Geometry check sheet. Reference: the model listing, model coordinates, mm. A direction names the side the tool comes from. Give positions to 0.01 mm unless a question says otherwise; leave off trailing zeros. Order: outer loops, then holes, each group sorted by start corner. A loop starts at its lowest first (then second) coordinate and runs counter-clockwise, first axis right, second up.
from build123d import *

# Parameters (mm, degrees)
SKETCH1_R                = 25
BOSS_EXTRUDE1_DEPTH      = 25
SKETCH9_W                = 25
SKETCH9_H                = 7.5
BOSS_EXTRUDE3_DEPTH      = 55
BOSS_EXTRUDE3_DEPTH_BACK = 55
SKETCH16_R               = 22.5
CUT_EXTRUDE3_DEPTH       = 7.5
SKETCH17_R               = 0.75
CUT_EXTRUDE4_DEPTH       = 10
SKETCH22_W               = 7.5
SKETCH22_H               = 25
BOSS_EXTRUDE7_DEPTH      = 30
SKETCH23_W               = 7.5
SKETCH23_H               = 60
BOSS_EXTRUDE8_DEPTH      = 110
SKETCH24_W               = 7.5
SKETCH24_H               = 80
BOSS_EXTRUDE9_DEPTH      = 110
SKETCH25_W               = 1.5
SKETCH25_H               = 110
BOSS_EXTRUDE10_DEPTH     = 2
SKETCH26_W               = 1.5
SKETCH26_H               = 110
BOSS_EXTRUDE11_DEPTH     = 2
FILLET6_R                = 5


with BuildPart() as part:
    # Sketch1 → Boss-Extrude1 (new body)
    with BuildSketch(Plane(origin=(0, 0, 0), x_dir=(1, 0, 0), z_dir=(0, 1, 0))):
        Circle(SKETCH1_R)
    extrude(amount=BOSS_EXTRUDE1_DEPTH)

    # Sketch9 → Boss-Extrude3 (add, two sides)
    with BuildSketch(Plane(origin=(0, 0, 0), x_dir=(0, 0, -1), z_dir=(1, 0, 0))) as boss_extrude3_sk:
        with Locations((0, 3.75)):
            Rectangle(SKETCH9_W, SKETCH9_H)
    extrude(amount=BOSS_EXTRUDE3_DEPTH)
    extrude(boss_extrude3_sk.sketch, amount=-BOSS_EXTRUDE3_DEPTH_BACK)

    # Sketch16 → Cut-Extrude3 (cut)
    with BuildSketch(Plane(origin=(0, 25, 0), x_dir=(1, 0, 0), z_dir=(0, 1, 0))):
        Circle(SKETCH16_R)
    extrude(amount=-CUT_EXTRUDE3_DEPTH, mode=Mode.SUBTRACT)

    # Sketch17 → Cut-Extrude4 (cut)
    with BuildSketch(Plane(origin=(0, 17.5, 0), x_dir=(1, 0, 0), z_dir=(0, 1, 0))):
        with BuildLine():
            ThreePointArc((-4, 3), (-3.535533906, 3.535533906), (-3, 4))
            Line((-3, 4), (-2, 22.410934831))
            ThreePointArc((-2, 22.410934831), (-15.909902577, 15.909902577), (-22.410934831, 2))
            Line((-22.410934831, 2), (-4, 3))
        make_face()
        with BuildLine():
            Line((2, 22.410934831), (3, 4))
            ThreePointArc((3, 4), (3.535533906, 3.535533906), (4, 3))
            Line((4, 3), (22.410934831, 2))
            ThreePointArc((22.410934831, 2), (15.909902577, 15.909902577), (2, 22.410934831))
        make_face()
        with BuildLine():
            ThreePointArc((-3, -4), (-3.535533906, -3.535533906), (-4, -3))
            Line((-4, -3), (-22.410934831, -2))
            ThreePointArc((-22.410934831, -2), (-15.909902577, -15.909902577), (-2, -22.410934831))
            Line((-2, -22.410934831), (-3, -4))
        make_face()
        with BuildLine():
            Line((22.410934831, -2), (4, -3))
            ThreePointArc((4, -3), (3.535533906, -3.535533906), (3, -4))
            Line((3, -4), (2, -22.410934831))
            ThreePointArc((2, -22.410934831), (15.909902577, -15.909902577), (22.410934831, -2))
        make_face()
        Circle(SKETCH17_R)
    extrude(amount=-CUT_EXTRUDE4_DEPTH, mode=Mode.SUBTRACT)

    # Sketch22 → Boss-Extrude7 (add)
    with BuildSketch(Plane.XZ):
        with Locations((-51.25, 0)):
            Rectangle(SKETCH22_W, SKETCH22_H)
    boss_extrude7 = extrude(amount=BOSS_EXTRUDE7_DEPTH)

    # Sketch23 → Boss-Extrude8 (add)
    with BuildSketch(Plane.XZ.offset(30)):
        with Locations((-51.25, 0)):
            Rectangle(SKETCH23_W, SKETCH23_H)
    extrude(amount=BOSS_EXTRUDE8_DEPTH)

    # Mirror1: Boss-Extrude7 across plane
    add(boss_extrude7.mirror(Plane(origin=(0, 0, 0), x_dir=(0, 0, 1), z_dir=(1, 0, 0))))

    # Sketch24 → Boss-Extrude9 (add)
    with BuildSketch(Plane.XZ.offset(30)):
        with Locations((51.25, 10)):
            Rectangle(SKETCH24_W, SKETCH24_H)
    extrude(amount=BOSS_EXTRUDE9_DEPTH)

    # Sketch25 → Boss-Extrude10 (add)
    with BuildSketch(Plane(origin=(-47.5, 0, 0), x_dir=(0, 0, -1), z_dir=(1, 0, 0))):
        with Locations((29.25, -85)):
            Rectangle(SKETCH25_W, SKETCH25_H)
    extrude(amount=BOSS_EXTRUDE10_DEPTH)

    # Sketch26 → Boss-Extrude11 (add)
    with BuildSketch(Plane.ZY.offset(-47.5)):
        with Locations((-29.25, -85)):
            Rectangle(SKETCH26_W, SKETCH26_H)
        with Locations((49.25, -85)):
            Rectangle(SKETCH26_W, SKETCH26_H)
    extrude(amount=BOSS_EXTRUDE11_DEPTH)

    # Fillet6
    fillet6_edges = [part.edges().sort_by_distance(p)[0] for p in [
        (-21.650635095, 3.75, 12.5),
        (21.650635095, 3.75, 12.5),
        (-55, 7.5, 0),
        (47.5, 0, 0),
        (21.650635095, 3.75, -12.5),
        (-21.650635095, 3.75, -12.5),
        (55, 7.5, 0),
        (-25, 7.5, 0),
        (-47.5, 0, 0),
        (24.148145657, 7.5, -6.470476128),
    ]]
    fillet(fillet6_edges, radius=FILLET6_R)


solid = part.part
Item 1: Scan lines: L1, parallel to X at y = -59, z = -1; L2, parallel to Z at x = 0, y = 12.75; L3, parallel to X at y = 10, z = 11. Record each from-to range of solid material in increasing order.
Reported:
L1: x = -55 to -47.5, 47.5 to 55
L2: z = -25 to -0.75, 0.75 to 25
L3: x = -23.19 to -19.63, -2.62 to 2.62, 19.63 to 23.19
Item 2: Sectioned sample at A-A (y = -77). Enter the section's corners in (x, z).
Reported:
outline: (-55, -30) - (-45.5, -30) - (-45.5, -28.5) - (-47.5, -28.5) - (-47.5, 30) - (-55, 30) - close; (45.5, -30) - (55, -30) - (55, 50) - (45.5, 50) - (45.5, 48.5) - (47.5, 48.5) - (47.5, -28.5) - (45.5, -28.5) - close
Item 3: Sectioned sample at D-D (y = 10). Enter the section's corners in (x, z), and give its area (3 significant figures).
Reported:
outline: (-22.11, -13.04) arc R5 cw to (-20.31, -14.58) arc R25 ccw to (20.31, -14.58) arc R5 cw to (22.11, -13.04) arc R25.67 ccw to (22.11, 13.04) arc R5 cw to (20.31, 14.58) arc R25 ccw to (-20.31, 14.58) arc R5 cw to (-22.11, 13.04) arc R25.67 ccw to start; hole (-22.41, -2) arc R22.5 ccw to (-2, -22.41) - (-3, -4) arc R5 cw to (-4, -3) - close; hole (-22.41, 2) - (-4, 3) arc R5 cw to (-3, 4) - (-2, 22.41) arc R22.5 ccw to start; hole circle Ø1.5 at (0, 0); hole (2, -22.41) arc R22.5 ccw to (22.41, -2) - (4, -3) arc R5 cw to (3, -4) - close; hole (2, 22.41) - (3, 4) arc R5 cw to (4, 3) - (22.41, 2) arc R22.5 ccw to start
area: 841 mm2
Item 4: Sectioned sample at B-B (x = 13.5). Enter the section's corners in (y, z), and give its area (3 significant figures).
Reported:
outline: (0, -21.04) - (25, -21.04) - (25, -18) - (7.5, -18) - (7.5, -2.48) - (17.5, -2.48) - (17.5, 2.48) - (7.5, 2.48) - (7.5, 18) - (25, 18) - (25, 21.04) - (0, 21.04) - close
area: 472 mm2
Item 5: Set-up check for faces 4 (the flat face through (-51, -84, 30)), 5 (the flat face through (2.493, 12.57, -13.334)), 6 (the flat face through (47, -2, -12.5)), 7 (the flat face through (-51, -30, -21)): record each of +Z, -Z, +X, -X, +Y, -Y from which the full face is reachable in a straight line by a thin tool's end or side.
Reported:
face 4: +Z, -X, +Y, -Y
face 5: +Y
face 6: -Z, +X, +Y
face 7: -Z, +X, -X, +Y
Item 6: Gauge pin test, flat ends, axial feed: pin 1 (6 mm diameter, centred on x = -49.5, z = 22, fed in from +Y); pin 2 (2 mm diameter, centred on x = -46, y = -89.5, fed in from +Z); pin 3 (6 mm diameter, centred on x = 16.5, z = 8, fed in from +Y). Record the tip position at first contact, or that the pin passes through.
Reported:
pin 1: stops at y = -30
pin 2: stops at z = -28.5
pin 3: stops at y = 7.5
Item 7: Sectioned sample at C-C (y = -23). Enter the section's corners in (x, z), and give its area (3 significant figures).
Reported:
outline: (-55, -12.5) - (-47.5, -12.5) - (-47.5, 12.5) - (-55, 12.5) - close; (47.5, -12.5) - (55, -12.5) - (55, 12.5) - (47.5, 12.5) - close
area: 375 mm2
Item 8: Draft check along Z on faces 1 (the flat face through (50, -84, 50)), 2 (the flat face through (-55, -84, 0)), 3 (the flat face through (-2.493, 12.57, 13.334)). Enter one of: released by +Z, released by -Z, zero draft, split by the parting line, or undercut.
Reported:
face 1: released by +Z
face 2: zero draft
face 3: undercut
